from build123d import *

# Parameters (mm, degrees)
SKETCH1_R           = 1.852456066
BOSS_EXTRUDE1_DEPTH = 4
CHAMFER1_SIZE       = 1


with BuildPart() as part:
    # Sketch1 → Boss-Extrude1 (new body)
    with BuildSketch(Plane(origin=(0, 0, 0), x_dir=(1, 0, 0), z_dir=(0, 1, 0))):
        with BuildLine():
            ThreePointArc((-4.845804171, 46.098557409), (0, 51.205005222), (4.845804171, 46.098557409))
            ThreePointArc((4.845804171, 46.098557409), (0, -46.352549156), (-4.845804171, 46.098557409))
        make_face()
        with Locations(Location((0, 46.352549156, 0), (0, 0, 270))):  # turned: the seam where the file's is
            Circle(SKETCH1_R, mode=Mode.SUBTRACT)
        with BuildLine():
            Line((-10.033402208, 9.809793399), (-13.883244786, -2.038803723))
            ThreePointArc((-13.883244786, -2.038803723), (-13.883244786, -4.510939678), (-12.43015973, -6.510939678))
            Line((-12.43015973, -6.510939678), (-2.351141009, -13.833775419))
            ThreePointArc((-2.351141009, -13.833775419), (0, -14.597707442), (2.351141009, -13.833775419))
            Line((2.351141009, -13.833775419), (12.43015973, -6.510939678))
            ThreePointArc((12.43015973, -6.510939678), (13.883244786, -4.510939678), (13.883244786, -2.038803723))
            Line((13.883244786, -2.038803723), (10.033402208, 9.809793399))
            ThreePointArc((10.033402208, 9.809793399), (8.580317152, 11.809793399), (6.229176142, 12.573725422))
            Line((6.229176142, 12.573725422), (-6.229176142, 12.573725422))
            ThreePointArc((-6.229176142, 12.573725422), (-8.580317152, 11.809793399), (-10.033402208, 9.809793399))
        make_face(mode=Mode.SUBTRACT)
        with BuildLine():
            Line((39.087870417, 8.530782914), (21.246938514, -4.431412853))
            ThreePointArc((21.246938514, -4.431412853), (19.793853458, -6.431412853), (19.793853458, -8.903548808))
            Line((19.793853458, -8.903548808), (26.608483054, -29.876822128))
            ThreePointArc((26.608483054, -29.876822128), (28.031122427, -31.200463964), (29.906376603, -30.69119756))
            ThreePointArc((29.906376603, -30.69119756), (40.755196115, -13.242165942), (42.234600213, 7.251173287))
            ThreePointArc((42.234600213, 7.251173287), (41.016826997, 8.765425211), (39.087870417, 8.530782914))
        make_face(mode=Mode.SUBTRACT)
        with BuildLine():
            Line((36.637019829, 16.073725422), (14.584415214, 16.073725422))
            ThreePointArc((14.584415214, 16.073725422), (12.233274205, 16.837657444), (10.780189149, 18.837657444))
            Line((10.780189149, 18.837657444), (3.965559553, 39.810930764))
            ThreePointArc((3.965559553, 39.810930764), (4.338481832, 41.717985947), (6.154933612, 42.40822752))
            ThreePointArc((6.154933612, 42.40822752), (25.188096417, 34.66844052), (38.430642043, 18.958552724))
            ThreePointArc((38.430642043, 18.958552724), (38.335497766, 17.017708046), (36.637019829, 16.073725422))
        make_face(mode=Mode.SUBTRACT)
        with BuildLine():
            Line((-3.965559553, 39.810930764), (-10.780189149, 18.837657444))
            ThreePointArc((-10.780189149, 18.837657444), (-12.233274205, 16.837657444), (-14.584415214, 16.073725422))
            Line((-14.584415214, 16.073725422), (-36.637019829, 16.073725422))
            ThreePointArc((-36.637019829, 16.073725422), (-38.335497766, 17.017708046), (-38.430642043, 18.958552724))
            ThreePointArc((-38.430642043, 18.958552724), (-25.188096417, 34.66844052), (-6.154933612, 42.40822752))
            ThreePointArc((-6.154933612, 42.40822752), (-4.338481832, 41.717985947), (-3.965559553, 39.810930764))
        make_face(mode=Mode.SUBTRACT)
        with BuildLine():
            Line((-39.087870417, 8.530782914), (-21.246938514, -4.431412853))
            ThreePointArc((-21.246938514, -4.431412853), (-19.793853458, -6.431412853), (-19.793853458, -8.903548808))
            Line((-19.793853458, -8.903548808), (-26.608483054, -29.876822128))
            ThreePointArc((-26.608483054, -29.876822128), (-28.031122427, -31.200463964), (-29.906376603, -30.69119756))
            ThreePointArc((-29.906376603, -30.69119756), (-40.755196115, -13.242165942), (-42.234600213, 7.251173287))
            ThreePointArc((-42.234600213, 7.251173287), (-41.016826997, 8.765425211), (-39.087870417, 8.530782914))
        make_face(mode=Mode.SUBTRACT)
        with BuildLine():
            Line((-20.192072912, -34.538616973), (-2.351141009, -21.576421206))
            ThreePointArc((-2.351141009, -21.576421206), (0, -20.812489183), (2.351141009, -21.576421206))
            Line((2.351141009, -21.576421206), (20.192072912, -34.538616973))
            ThreePointArc((20.192072912, -34.538616973), (21.011311363, -36.30065524), (19.947484821, -37.926755971))
            ThreePointArc((19.947484821, -37.926755971), (0, -42.852549156), (-19.947484821, -37.926755971))
            ThreePointArc((-19.947484821, -37.926755971), (-21.011311363, -36.30065524), (-20.192072912, -34.538616973))
        make_face(mode=Mode.SUBTRACT)
        with BuildLine():
            Line((-15.56822788, 12.573725422), (-35.620264195, 12.573725422))
            ThreePointArc((-35.620264195, 12.573725422), (-36.571320711, 11.882742416), (-36.208049447, 10.764708428))
            Line((-36.208049447, 10.764708428), (-19.985611297, -1.021582797))
            ThreePointArc((-19.985611297, -1.021582797), (-18.192006803, -1.30566184), (-16.90792776, -0.021582797))
            Line((-16.90792776, -0.021582797), (-13.666114848, 9.955691433))
            ThreePointArc((-13.666114848, 9.955691433), (-13.950193891, 11.749295926), (-15.56822788, 12.573725422))
        make_face(mode=Mode.SUBTRACT)
        with BuildLine():
            Line((-7.147476509, 18.691759411), (-0.951056516, 37.762379212))
            ThreePointArc((-0.951056516, 37.762379212), (0, 38.453362218), (0.951056516, 37.762379212))
            Line((0.951056516, 37.762379212), (7.147476509, 18.691759411))
            ThreePointArc((7.147476509, 18.691759411), (6.863397465, 16.898154917), (5.245363477, 16.073725422))
            Line((5.245363477, 16.073725422), (-5.245363477, 16.073725422))
            ThreePointArc((-5.245363477, 16.073725422), (-6.863397465, 16.898154917), (-7.147476509, 18.691759411))
        make_face(mode=Mode.SUBTRACT)
        with BuildLine():
            Line((15.56822788, 12.573725422), (35.620264195, 12.573725422))
            ThreePointArc((35.620264195, 12.573725422), (36.571320711, 11.882742416), (36.208049447, 10.764708428))
            Line((36.208049447, 10.764708428), (19.985611297, -1.021582797))
            ThreePointArc((19.985611297, -1.021582797), (18.192006803, -1.30566184), (16.90792776, -0.021582797))
            Line((16.90792776, -0.021582797), (13.666114848, 9.955691433))
            ThreePointArc((13.666114848, 9.955691433), (13.950193891, 11.749295926), (15.56822788, 12.573725422))
        make_face(mode=Mode.SUBTRACT)
        with BuildLine():
            Line((22.965590477, -29.991389537), (16.769170484, -10.920769735))
            ThreePointArc((16.769170484, -10.920769735), (15.48509144, -9.636690691), (13.691486947, -9.920769735))
            Line((13.691486947, -9.920769735), (5.204310558, -16.087064324))
            ThreePointArc((5.204310558, -16.087064324), (4.379881063, -17.705098312), (5.204310558, -19.323132301))
            Line((5.204310558, -19.323132301), (21.426748708, -31.109423525))
            ThreePointArc((21.426748708, -31.109423525), (22.602319213, -31.109423525), (22.965590477, -29.991389537))
        make_face(mode=Mode.SUBTRACT)
        with BuildLine():
            Line((-22.965590477, -29.991389537), (-16.769170484, -10.920769735))
            ThreePointArc((-16.769170484, -10.920769735), (-15.48509144, -9.636690691), (-13.691486947, -9.920769735))
            Line((-13.691486947, -9.920769735), (-5.204310558, -16.087064324))
            ThreePointArc((-5.204310558, -16.087064324), (-4.379881063, -17.705098312), (-5.204310558, -19.323132301))
            Line((-5.204310558, -19.323132301), (-21.426748708, -31.109423525))
            ThreePointArc((-21.426748708, -31.109423525), (-22.602319213, -31.109423525), (-22.965590477, -29.991389537))
        make_face(mode=Mode.SUBTRACT)
    extrude(amount=BOSS_EXTRUDE1_DEPTH)

    # Chamfer1
    chamfer1_edges = [part.edges().sort_by_distance(p)[0] for p in [
        (21.011311363, 4, 36.30065524),
        (11.271606961, 4, 28.057519089),
        (-19.793853458, 4, 6.431412853),
        (-30.167404466, 4, -2.049685031),
        (-41.016826997, 4, -8.765425211),
        (-40.755196115, 4, 13.242165942),
        (-28.031122427, 4, 31.200463964),
        (-23.201168256, 4, 19.390185468),
        (-18.192006803, 4, 1.30566184),
        (-15.287021304, 4, -4.967054318),
        (-13.950193891, 4, -11.749295926),
        (-25.594246037, 4, -12.573725422),
        (-36.571320711, 4, -11.882742416),
        (-28.096830372, 4, -4.871562815),
        (-6.863397465, 4, -16.898154917),
        (0, 4, -16.073725422),
        (6.863397465, 4, -16.898154917),
        (4.049266513, 4, -28.227069312),
        (0, 4, -38.453362218),
        (-4.049266513, 4, -28.227069312),
        (13.950193891, 4, -11.749295926),
        (15.287021304, 4, -4.967054318),
        (18.192006803, 4, 1.30566184),
        (28.096830372, 4, -4.871562815),
        (36.571320711, 4, -11.882742416),
        (25.594246037, 4, -12.573725422),
        (15.48509144, 4, 9.636690691),
        (9.447898752, 4, 13.003917029),
        (4.379881063, 4, 17.705098312),
        (13.315529633, 4, 25.216277913),
        (-13.883244786, 4, 4.510939678),
        (22.602319213, 4, 31.109423525),
        (19.86738048, 4, 20.456079636),
        (-7.390650369, 4, 10.172357549),
        (0, 4, 14.597707442),
        (7.390650369, 4, 10.172357549),
        (13.883244786, 4, 4.510939678),
        (11.958323497, 4, -3.885494838),
        (-4.379881063, 4, 17.705098312),
        (-9.447898752, 4, 13.003917029),
        (-15.48509144, 4, 9.636690691),
        (8.580317152, 4, -11.809793399),
        (-19.86738048, 4, 20.456079636),
        (-22.602319213, 4, 31.109423525),
        (-13.315529633, 4, 25.216277913),
        (0, 4, -12.573725422),
        (-8.580317152, 4, -11.809793399),
        (-11.958323497, 4, -3.885494838),
        (0, 4, -48.205005222),
        (0, 4, 46.352549156),
        (-12.233274205, 4, -16.837657444),
        (-7.372874351, 4, -29.324294104),
        (-4.338481832, 4, -41.717985947),
        (-25.188096417, 4, -34.66844052),
        (-38.335497766, 4, -17.017708046),
        (-25.610717522, 4, -16.073725422),
        (12.233274205, 4, -16.837657444),
        (25.610717522, 4, -16.073725422),
        (38.335497766, 4, -17.017708046),
        (25.188096417, 4, -34.66844052),
        (4.338481832, 4, -41.717985947),
        (7.372874351, 4, -29.324294104),
        (0, 4, -51.205005222),
        (19.793853458, 4, 6.431412853),
        (23.201168256, 4, 19.390185468),
        (28.031122427, 4, 31.200463964),
        (40.755196115, 4, 13.242165942),
        (41.016826997, 4, -8.765425211),
        (30.167404466, 4, -2.049685031),
        (0, 4, 20.812489183),
        (-11.271606961, 4, 28.057519089),
        (-21.011311363, 4, 36.30065524),
        (0, 4, 42.852549156),
    ]]
    chamfer(chamfer1_edges, length=CHAMFER1_SIZE)


solid = part.part
The listing builds one solid part. Answer for the finished solid, in the listing's coordinates (mm). A direction names the side the tool comes from. Round coordinates to 2 decimals unless told otherwise and drop trailing zeros. Write each question's results on one line, items separated by ' | '. Start each with the question number.
(1) For faces 1 (the flat face through (-6.84, 3.51, -29.31)), 2 (the cylindrical face through (28.004, 1.479, 31.193)), determine the directions among +Z, -Z, +X, -X, +Y, -Y from which every point of the face is accessible in a straight line to the end or side of a thin tool.
(2) Find the intervals of material crossed by line 1 (X direction, y = 0.6, z = -21); line 2 (X direction, y = 0.4, z = 27); line 3 (Z direction, x = -33.5, y = 2), in increasing order.
(3) The part is cut by section A-A, the plane y = 1.15. Give the number of separate pieces and of enclosed holes in the cut face, and give its area (3 significant figures).
(4) Each of these flat-tipped pins is pushed along its axis until it touches: P1, Ø0.9, axis at x = 30, y = 2, coming from the -Z side; P2, Ø0.9, axis at x = -23.5, y = 1.5, coming from the +Z side; P3, Ø1.5, axis at x = 28.5, y = 0.5, coming from the +Z side. Where does it stop, or does it pass through?
Worked answers:
1) face 1: +Y | face 2: +Y, -Y
2) line 1: x = -41.32 to -37.35, -10.08 to -6.4, 6.4 to 10.08, 37.35 to 41.32 | line 2: x = -37.68 to -33.28, -25.67 to -21.99, -15.77 to -9.82, 9.82 to 15.77, 21.99 to 25.67, 33.28 to 37.68 | line 3: z = -32.04 to -26.72, -16.07 to -12.57, -8.8 to -4.47, 26.72 to 32.04
3) separate pieces: 1 | enclosed holes: 12 | area: 2,410 mm²
4) P1: stops at z = -35.71 | P2: stops at z = 40.22 | P3: stops at z = 37.13
